Geometry check sheet. Reference: drawing and pictorial views, mm from the part's lowest x, y, z. A direction names the side the tool comes from. Round coordinates to 2 decimals unless told otherwise and drop trailing zeros. Loops run counter-clockwise (first coordinate to the right, second up) from the corner with the lowest first, then second, coordinate; pieces in that order, holes last. Notation, with made-up numbers: (-29, 26) - (12, 26) arc R21 cw to (12, 52) - close; hole circle Ø7 at (-10.75, -39.5). An arc over 180 degrees is marked (long way). Return JSON: item names as keys, results as strings.
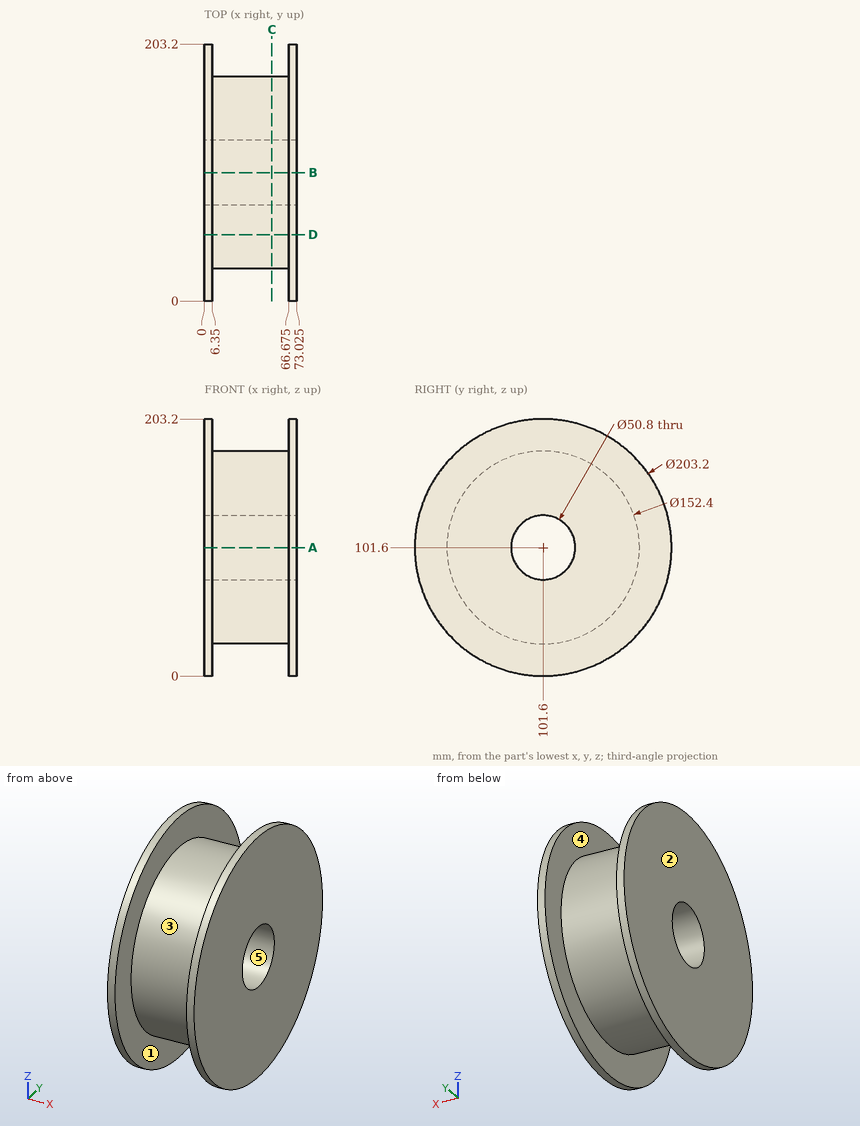
Q1. Draft check along Y on the marked faces 3, 4 and 5. Enter one of: released by +Y, released by -Y, zero draft, split by the parting line, or undercut.
Answer key:
{"face 3": "split by the parting line", "face 4": "zero draft", "face 5": "undercut"}
Q2. Tool access check on the marked faces 1 and 2. Record the directions out of +Z, -Z, +X, -X, +Y, -Y that give a thin tool (end or side, any length) a straight path to the whole face; none if there is none.
Answer key:
{"face 1": "none", "face 2": "+Z, -Z, -X, +Y, -Y"}
Q3. Sectioned sample at D-D (y = 52.5). Enter the section's corners in (x, z) (3 decimals).
Answer key:
{"outline": "(0, 12.652) - (6.35, 12.652) - (6.35, 43.328) - (66.675, 43.328) - (66.675, 12.652) - (73.025, 12.652) - (73.025, 190.548) - (66.675, 190.548) - (66.675, 159.872) - (6.35, 159.872) - (6.35, 190.548) - (0, 190.548) - close"}
Q4. Sectioned sample at A-A (z = 101.6). Enter the section's corners in (x, y) (3 decimals), plus the area to 3 significant figures.
Answer key:
{"outline": "(0, 0) - (6.35, 0) - (6.35, 25.4) - (66.675, 25.4) - (66.675, 0) - (73.025, 0) - (73.025, 76.2) - (0, 76.2) - close; (0, 127) - (73.025, 127) - (73.025, 203.2) - (66.675, 203.2) - (66.675, 177.8) - (6.35, 177.8) - (6.35, 203.2) - (0, 203.2) - close", "area": "8,060 mm²"}
Q5. Sectioned sample at C-C (x = 53.5). Enter the section's corners in (y, z).
Answer key:
{"outline": "circle Ø152.4 at (101.6, 101.6); hole circle Ø50.8 at (101.6, 101.6)"}
Q6. Scan lines: probe 1 along Z at (x, y) = (49.5, 101.6); probe 2 along X at (y, z) = (62.5, 8.5) (3 decimals); probe 3 along Y at (x, z) = (17, 101). Record each from-to range of solid material in increasing order. Write a range as [from, to].
Answer key:
{"probe 1": "z = [25.4, 76.2], [127, 177.8]", "probe 2": "x = [0, 6.35], [66.675, 73.025]", "probe 3": "y = [25.4, 76.21], [126.99, 177.8]"}
Q7. Depth check by flat-ended pin: P1, Ø12, axis at x = 25, z = 150, coming from the -Y side; P2, Ø12, axis at x = 57.5, z = 178, coming from the -Y side; P3, Ø3, axis at x = 15.5, y = 65, coming from the +Z side. Enter the tip coordinate at first touch or a pass-through.
Answer key:
{"P1": "stops at y = 38.29", "P2": "stops at y = 72.44", "P3": "stops at z = 169.23"}
